```python
from build123d import *

# Parameters (mm, degrees)
SKETCH001_R = 2.5
PAD_DEPTH   = 3


with BuildPart() as part:
    # Sketch001 → Pad (new body)
    with BuildSketch(Plane(origin=(0, 0, 0), x_dir=(1, 0, 0), z_dir=(0, 0, -1))):
        with BuildLine():
            ThreePointArc((45.02147, 90.410548), (36.084716, 99.82444), (35.972243, 86.844676))
            ThreePointArc((86.844676, 35.972243), (66.468037, 66.468037), (35.972243, 86.844676))
            ThreePointArc((86.844676, 35.972243), (99.82444, 36.084716), (90.410548, 45.02147))
            ThreePointArc((90.410548, 45.02147), (71.417785, 71.417785), (45.02147, 90.410548))
        make_face()
        with Locations((38.651027, 93.311833)):
            Circle(SKETCH001_R, mode=Mode.SUBTRACT)
        with Locations((93.311833, 38.651027)):
            Circle(SKETCH001_R, mode=Mode.SUBTRACT)
    extrude(amount=PAD_DEPTH)


solid = part.part
```
Here's how the part is built. I have some questions about the finished solid (model axes, mm). Give positions to 0.01 mm unless a question says otherwise; leave off trailing zeros. Write each loop counter-clockwise with the first axis right and the second up, starting at its lowest first coordinate (ties: lowest second). Pieces come first, ordered by that corner, then holes. Notation, with made-up numbers: M 3,74.25 L 14,74.25 A35 ccw 14,109.25 Z; hole C -37.5,61.5 d3. An arc over 180 degrees is marked long. Put each result on its own line as item: value. Start each with the question number.
Item 1: If we section it at D-D, the plane y = -89.5: Write out the boundary of the cut face in (x, z), then the cut area to 3 significant figures.
Item 2: If we section it at B-B, the plane x = 94: Write out the boundary of the cut face in (y, z).
Item 3: Will these pins go through, and if not, where does the flat tip stop? pin 1 (1.5 mm diameter, centred on x = 47, z = -2, fed in from -Y); pin 2 (1.5 mm diameter, centred on x = 54, z = -2.5, fed in from -Y); pin 3 (3 mm diameter, centred on x = 38.65, y = -93.31, fed in from +Z); pin 4 (1.5 mm diameter, centred on x = 38.5, z = -2.5, fed in from +Y).
Item 4: I need wall thicknesses on L1, parallel to X at y = -37.5, z = -1.3; L2, parallel to Y at x = 39, z = -2.65; L3, parallel to Y at x = 36.5, z = -0.4. Which ranges of each line are inside material? Lowest first, please. Write a range as from..to.
Item 5: Thinking about a two-plate mould opening in X: for faces 1 (the cylindrical face through (38.11, -90.87, -1.48)), 2 (the flat face through (66, -69, -3)), 3 (the cylindrical face through (36.303, -99.906, -1.479)), which applies, +X half, -X half, draft (parallel to the pull), parting line (faces both ways), or undercut?
Item 6: If we section it at C-C, the plane z = -2.3: Write out the boundary of the cut face in (x, y), then the cut area to 3 significant figures.
Item 7: If we section it at A-A, the plane y = -37: Write out the boundary of the cut face in (x, z), then the cut area to 3 significant figures.
Values:
1. outline: M 32.78,-3 L 46.81,-3 L 46.81,0 L 32.78,0 Z
1. area: 42.1 mm²
2. outline: M -45.62,-3 L -41.05,-3 L -41.05,0 L -45.62,0 Z; M -36.25,-3 L -31.68,-3 L -31.68,0 L -36.25,0 Z
3. pin 1: y = -89.79
3. pin 2: y = -85.82
3. pin 3: through
3. pin 4: y = -85.41
4. L1: 86.2..91.09, 95.53..100.22
4. L2: -100.3..-95.79, -90.84..-85.53
4. L3: -99.97..-94.59, -92.04..-86.62
5. face 1: undercut
5. face 2: draft
5. face 3: parting line
6. outline: M 35.97,-86.84 A7 ccw long 45.02,-90.41 A101 ccw 90.41,-45.02 A7 ccw long 86.84,-35.97 A94 cw Z; hole C 38.65,-93.31 d5; hole C 93.31,-38.65 d5
6. area: 729 mm²
7. outline: M 86.41,-3 L 91.43,-3 L 91.43,0 L 86.41,0 Z; M 95.19,-3 L 100.11,-3 L 100.11,0 L 95.19,0 Z
7. area: 29.8 mm²
